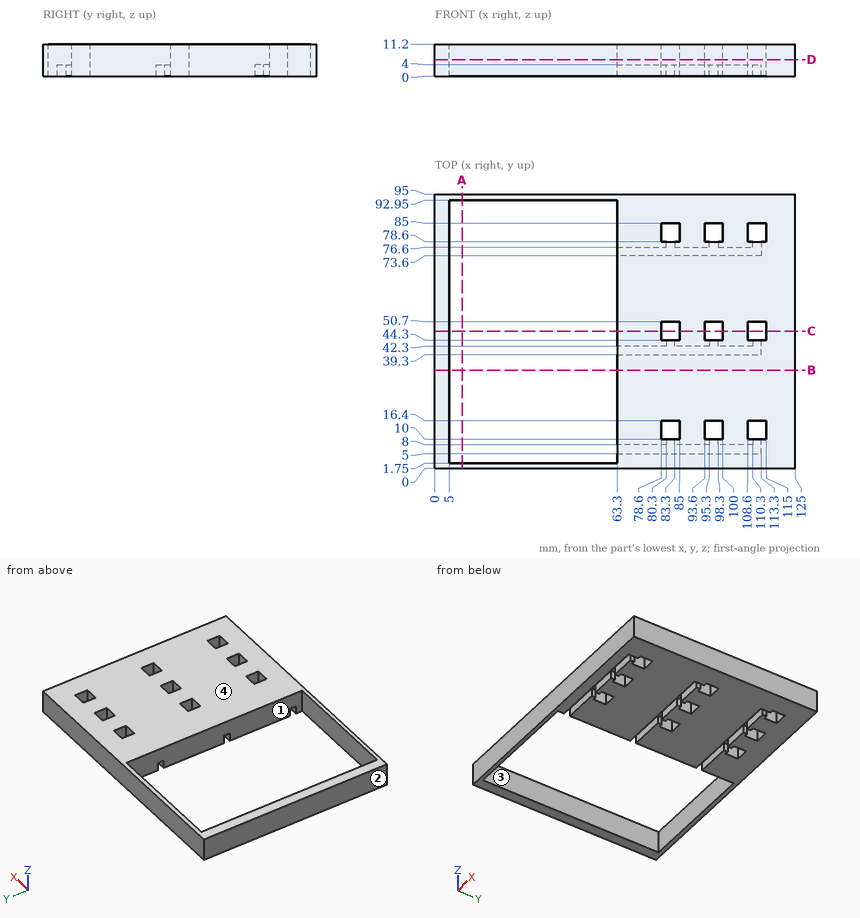
Source: three-view drawing plus pictorial views. Frame: mm from the lowest corner of the part. A direction names the side the tool comes from. Give positions to 0.01 mm unless a question says otherwise; leave off trailing zeros. Order: outer loops, then holes, each group sorted by start corner. A loop starts at its lowest first (then second) coordinate and runs counter-clockwise, first axis right, second up. Notation, with made-up numbers: (-20.5, -13) -> (34.5, -13) arc R32 ccw to (34.5, 22) -> close; hole circle Ø7 at (-37, 81). An arc over 180 degrees is marked (long way). Put each result on its own line as item: value.
Q1. Section B-B, the plane y = 34. Return loops of the section in (x, z), then the cut area to 3 significant figures.
Here are the results:
outline: (0, 0) -> (5, 0) -> (5, 11.2) -> (0, 11.2) -> close; (63.3, 0) -> (125, 0) -> (125, 11.2) -> (63.3, 11.2) -> close
area: 747 mm^2
Q2. Section A-A, the plane x = 9.5. Return loops of the section in (y, z).
Here are the results:
outline: (0, 0) -> (1.75, 0) -> (1.75, 11.2) -> (0, 11.2) -> close; (92.95, 0) -> (95, 0) -> (95, 11.2) -> (92.95, 11.2) -> close
Q3. Draft query along Y for the marked faces 1 and 2. Return one class per face: released by +Y, released by -Y, zero draft, split by the parting line, or undercut.
Here are the results:
face 1: undercut
face 2: zero draft
Q4. Material intervals for L1, parallel to Y at x = 72, z = 2.25; L2, parallel to X at y = 11, z = 3; L3, parallel to Y at x = 113, z = 5, sorted ascending.
Here are the results:
L1: y = 0 to 5, 8 to 39.3, 42.3 to 73.6, 76.6 to 95
L2: x = 0 to 5, 63.3 to 78.6, 85 to 93.6, 100 to 108.6, 115 to 125
L3: y = 0 to 10, 16.4 to 44.3, 50.7 to 78.6, 85 to 95
Q5. Section C-C, the plane y = 47.5. Return loops of the section in (x, z), then the cut area to 3 significant figures.
Here are the results:
outline: (0, 0) -> (5, 0) -> (5, 11.2) -> (0, 11.2) -> close; (63.3, 0) -> (78.6, 0) -> (78.6, 11.2) -> (63.3, 11.2) -> close; (85, 0) -> (93.6, 0) -> (93.6, 11.2) -> (85, 11.2) -> close; (100, 0) -> (108.6, 0) -> (108.6, 11.2) -> (100, 11.2) -> close; (115, 0) -> (125, 0) -> (125, 11.2) -> (115, 11.2) -> close
area: 532 mm^2
Q6. Section D-D, the plane z = 5.75. Count the separate pieces of the cut face and the enclosed holes in it, then the cut area to 3 significant figures.
Here are the results:
separate pieces: 1
enclosed holes: 10
area: 6,190 mm^2
Q7. Reachability of the marked faces 3 and 4 from +Z, -Z, +X, -X, +Y, -Y: full face, straight path, thin tool, end or side. Return the list, or none.
Here are the results:
face 3: +Z, -Z
face 4: +Z, +X, -X, +Y, -Y
